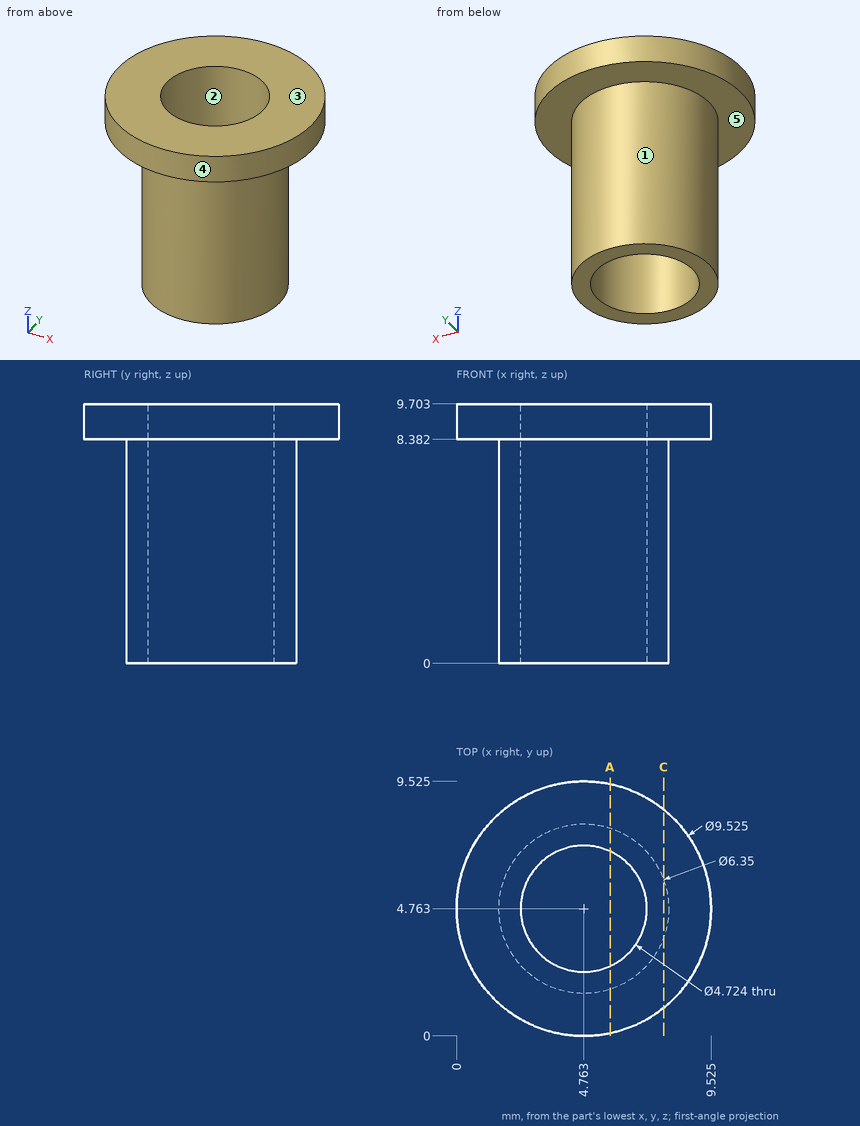
Design review of the part shown in the three views and the two pictorial views. Dimensions are in mm from the part's minimum x, y and z. A direction names the side the tool comes from. Round coordinates to 2 decimals unless told otherwise and drop trailing zeros. Write each loop counter-clockwise with the first axis right and the second up, starting at its lowest first coordinate (ties: lowest second). Pieces come first, ordered by that corner, then holes. Notation, with made-up numbers: (83.5, 60) - (117.5, 60) arc R21 ccw to (117.5, 89) - close; hole circle Ø4 at (-36.5, 72). An arc over 180 degrees is marked (long way). Write item = value, one per line. Start each with the question number.
1. Draft analysis for pull direction Y (two halves, no side actions). For the marked faces 1, 2 and 3, state which applies: released by +Y, released by -Y, zero draft, split by the parting line, or undercut.
2. Consider section C-C on x = 7.75. State the section outline as (y, z) points.
3. For pin 1 Ø1 at (x, z) = (8, 7.5) entering from -Y (1 decimal); pin 2 Ø1 at (x, z) = (6.5, 5.5) entering from +Y; pin 3 Ø3 at (x, z) = (6.5, 4.5) entering from -Y, all flat-tipped, find the tip position at first contact; note any pin that passes through.
4. Consider section A-A on x = 5.75. State the section outline as (y, z) points (1 decimal).
5. Wall thickness on L1, parallel to Y at x = 4.75, z = 8.75 (1 decimal); L2, parallel to X at y = 4.75, z = 4.5 (1 decimal); L3, parallel to Z at x = 6.25, y = 1.75: over which ranges is each line inside the solid? List them lowest first.
6. For the marked faces 4 and 5, list the 3-axis set-ups (+Z, -Z, +X, -X, +Y, -Y) from which the entire face can be reached by the end or side of a thin tool; tool diameter is ignored.
Evaluation:
q1.face_1 = split by the parting line
q1.face_2 = undercut
q1.face_3 = zero draft
q2.outline = (1.05, 8.38) - (3.69, 8.38) - (3.69, 0) - (5.84, 0) - (5.84, 8.38) - (8.47, 8.38) - (8.47, 9.7) - (1.05, 9.7) - close
q3.pin_1 = 3.2
q3.pin_2 = 7.69
q3.pin_3 = 1.6
q4.outline = (0.1, 8.4) - (1.7, 8.4) - (1.7, 0) - (2.6, 0) - (2.6, 9.7) - (0.1, 9.7) - close; (6.9, 0) - (7.8, 0) - (7.8, 8.4) - (9.4, 8.4) - (9.4, 9.7) - (6.9, 9.7) - close
q5.L1 = 0 to 2.4, 7.1 to 9.5
q5.L2 = 1.6 to 2.4, 7.1 to 7.9
q5.L3 = 8.38 to 9.7
q6.face_4 = +Z, -Z
q6.face_5 = -Z
